from build123d import *

# Parameters (mm, degrees)
SKETCH1_W           = 136.711090248
SKETCH1_H           = 77.79453909
BOSS_EXTRUDE1_DEPTH = 10
SKETCH2_R           = 2.416271905
CUT_EXTRUDE1_DEPTH  = 10
SKETCH3_R           = 4.303274805
CUT_EXTRUDE2_DEPTH  = 3


with BuildPart() as part:
    # Sketch1 → Boss-Extrude1 (new body)
    with BuildSketch(Plane(origin=(0, 0, 0), x_dir=(1, 0, 0), z_dir=(0, 1, 0))):
        Rectangle(SKETCH1_W, SKETCH1_H)
    extrude(amount=BOSS_EXTRUDE1_DEPTH)

    # Sketch2 → Cut-Extrude1 (cut)
    with BuildSketch(Plane(origin=(0, 10, 0), x_dir=(1, 0, 0), z_dir=(0, 1, 0))):
        with Locations(Location((-49.353103883, 25.56048813, 0), (0, 0, 270))):
            Circle(SKETCH2_R)
    cut_extrude1 = extrude(amount=-CUT_EXTRUDE1_DEPTH, mode=Mode.SUBTRACT)

    # Sketch3 → Cut-Extrude2 (cut)
    with BuildSketch(Plane(origin=(0, 10, 0), x_dir=(1, 0, 0), z_dir=(0, 1, 0))):
        with Locations(Location((-49.353103883, 25.56048813, 0), (0, 0, 270))):
            Circle(SKETCH3_R)
    cut_extrude2 = extrude(amount=-CUT_EXTRUDE2_DEPTH, mode=Mode.SUBTRACT)

    # Sketch-Pattern1: Cut-Extrude1, Cut-Extrude2 at 9 more places
    with Locations((71.598831, 0, 5.745585), (72.63009, 0, 38.74587), (28.727926, 0, -1.62055), (-2.946454, 0, 23.571632), (18.268015, 0, 46.995941), (97.822272, 0, -1.031259), (108.576829, 0, 35.799416), (28.580603, 0, 22.39305), (55.68798, 0, 50.384363)):
        add(cut_extrude1, mode=Mode.SUBTRACT)
        add(cut_extrude2, mode=Mode.SUBTRACT)


solid = part.part
CAD build for the part. Positions are in the model's coordinates, mm. A direction names the side the tool comes from. Give positions to 0.01 mm unless a question says otherwise; leave off trailing zeros. Write each question's results on one line, items separated by ' | '.
Q1. Flat gauge pins, fed straight in: P1, Ø4, axis at x = 18.5, z = -4.5, coming from the -Y side; P2, Ø4.5, axis at x = -33, z = 21, coming from the +Y side. Where does each tip first touch, or does it go through?
Geometry check:
P1: stops at y = 0 | P2: stops at y = 7
Q2. Band-saw the part on A-A on y = 4.75. Give the number of separate pieces and of enclosed holes in the cut face, and give its area (3 significant figures).
Geometry check:
separate pieces: 1 | enclosed holes: 10 | area: 10,500 mm²
Q3. Mould opens along X. For faces 3 (the face through (-54.66, 3.55, -2.51)), 4 (the face through (-1, 0, -1)), 5 (the face through (68.356, 5, 1)) say: pulls with the +X half, pulls with the -X half, needs draft (parallel to the pull), parting line crosses it, or undercut.
Geometry check:
face 3: undercut | face 4: needs draft | face 5: pulls with the +X half
Q4. Which spindle directions (+Z, -Z, +X, -X, +Y, -Y) get a long thin tool onto all of the face, cutting with end or side? Do faces 1 (the face through (-32.9, 7, 23.3)), 2 (the face through (-1, 5, 38.897)). Say none if no direction does.
Geometry check:
face 1: +Y | face 2: +Z, +X, -X, +Y, -Y
Q5. Probe probe 1 along X at (y, z) = (3, 21.5); probe 2 along X at (y, z) = (2.75, 11.5); probe 3 along Z at (x, y) = (-20, 6). List the from-to ranges inside material, lowest first.
Geometry check:
probe 1: x = -68.36 to -33.5, -28.67 to 68.36 | probe 2: x = -68.36 to 21.55, 25.01 to 57.16, 61.28 to 68.36 | probe 3: z = -38.9 to -29.52, -24.85 to -5.46, -0.88 to 38.9
